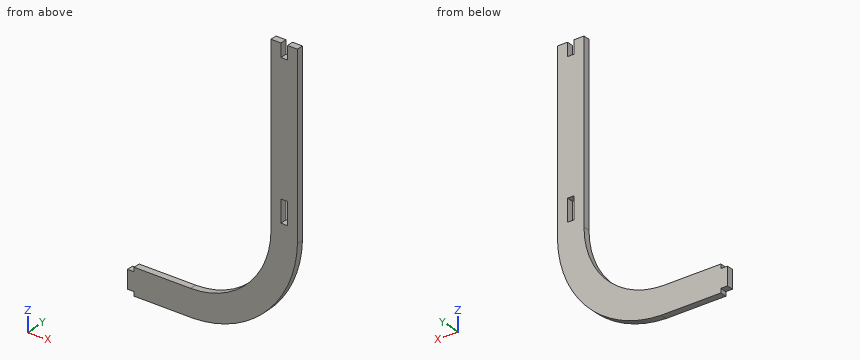
from build123d import *

# Parameters (mm, degrees)
SALIENTE_EXTRUIR1_DEPTH = 3


with BuildPart() as part:
    # Croquis1 → Saliente-Extruir1 (new body)
    with BuildSketch(Plane(origin=(0, 0, 0), x_dir=(1, 0, 0), z_dir=(0, 1, 0))):
        with BuildLine():
            Line((0, 7.786096257), (0, 0))
            Line((0, 0), (0, -0.213903743))
            Line((0, -0.213903743), (3, -0.213903743))
            Line((3, -0.213903743), (3, -2.106951872))
            Line((3, -2.106951872), (7.35828877, -2.106951872))
            Line((7.35828877, -2.106951872), (28.573593129, -2.106951872))
            ThreePointArc((28.573593129, -2.106951872), (54.330952442, -12.77599943), (65, -38.533358743))
            Line((65, -38.533358743), (65, -117.736951872))
            Line((65, -117.736951872), (69.5, -117.736951872))
            Line((69.5, -117.736951872), (69.5, -111.736951872))
            Line((69.5, -111.736951872), (72.5, -111.736951872))
            Line((72.5, -111.736951872), (72.5, -117.736951872))
            Line((72.5, -117.736951872), (77, -117.736951872))
            Line((77, -117.736951872), (77, -37.153707926))
            ThreePointArc((77, -37.153707926), (62.830127679, -4.276824192), (29.953243946, 9.893048128))
            Line((29.953243946, 9.893048128), (7.35828877, 9.893048128))
            Line((7.35828877, 9.893048128), (3, 9.893048128))
            Line((3, 9.893048128), (3, 8))
            Line((3, 8), (0, 8))
            Line((0, 8), (0, 7.786096257))
        make_face()
        Polygon((69.5, -53.106951872), (69.5, -48.106951872), (69.5, -43.106951872), (72.5, -43.106951872), (72.5, -53.106951872), align=None, mode=Mode.SUBTRACT)
    extrude(amount=SALIENTE_EXTRUIR1_DEPTH)


solid = part.part
Design review of the part built by this model. Coordinates are the model's own, in mm. Give positions to 0.01 mm unless a question says otherwise; leave off trailing zeros. Write each loop counter-clockwise with the first axis right and the second up, starting at its lowest first coordinate (ties: lowest second). Pieces come first, ordered by that corner, then holes. Notation, with made-up numbers: M 78,57.25 L 82,57.25 A7 ccw 82,61.25 Z; hole C 18.5,-11.5 d5. An arc over 180 degrees is marked long. Return JSON: item names as keys, results as strings. Group by question number.
Item 1: Wall thickness on line 1 along X through (y, z) = (1.9, 45); line 2 along X through (y, z) = (2.25, 57); line 3 along Z through (x, y) = (12, 1.9): over which ranges is each line inside the solid? List them lowest first.
Item 2: Clearance check with flat-ended pins moving along their axes: pin 1 Ø1.5 at (y, z) = (1.5, 1) entering from -X; pin 2 Ø1.5 at (y, z) = (1, 116) entering from -X; pin 3 Ø1.5 at (x, y) = (35, 1) entering from +Z. State where each tip first meets the part, or that it passes through.
Item 3: Take a section at B-B (z = 95.5). Give the boundary of the cut face in (x, y), plus the area to 3 significant figures.
Item 4: Take a section at A-A (y = 1.5). Give the boundary of the cut face in (x, z).
Item 5: Take a section at C-C (x = 8). Give the boundary of the cut face in (y, z).
Return value:
{
 "1": {"line 1": "x = 65 to 69.5, 72.5 to 77", "line 2": "x = 65 to 77", "line 3": "z = -9.89 to 2.11"},
 "2": {"pin 1": "stops at x = 3", "pin 2": "stops at x = 65", "pin 3": "stops at z = 2.82"},
 "3": {"outline": "M 65,0 L 77,0 L 77,3 L 65,3 Z", "area": "36.0 mm2"},
 "4": {"outline": "M 0,-8 L 3,-8 L 3,-9.89 L 29.95,-9.89 A48.45 ccw 77,37.15 L 77,117.74 L 72.5,117.74 L 72.5,111.74 L 69.5,111.74 L 69.5,117.74 L 65,117.74 L 65,38.53 A36.43 cw 28.57,2.11 L 3,2.11 L 3,0.21 L 0,0.21 Z; hole M 69.5,43.11 L 72.5,43.11 L 72.5,53.11 L 69.5,53.11 Z"},
 "5": {"outline": "M 0,-9.89 L 3,-9.89 L 3,2.11 L 0,2.11 Z"}
}
